from build123d import *

# Parameters (mm, degrees)
SCHNITT_LINEAR_AUSTRAGEN2_DEPTH = 7.5


with BuildPart() as part:
    # Skizze1 → Rotation1 (revolve)
    with BuildSketch(Plane.XY, mode=Mode.PRIVATE) as rotation1_sk:
        with BuildLine():
            Line((14.3, 4.8), (15.4, 4.8))
            Line((15.4, 4.8), (15.4, 5))
            Line((15.4, 5), (16.4, 5))
            Line((16.4, 5), (16.9, 4.5))
            Line((16.9, 4.5), (16.9, 0))
            Line((16.9, 0), (-12.3, 0))
            Line((-12.3, 0), (-12.3, 5))
            Line((-12.3, 5), (-3.05, 5))
            Line((-3.05, 5), (-3.05, 4.25))
            Line((-3.05, 4.25), (-2.3, 4.25))
            Line((-2.3, 4.25), (-2.3, 7.5))
            Line((-2.3, 7.5), (-0.7, 7.5))
            Line((-0.7, 7.5), (-0.7, 5.3))
            ThreePointArc((-0.7, 5.3), (-0.612132034, 5.087867966), (-0.4, 5))
            Line((-0.4, 5), (14.3, 5))
            Line((14.3, 5), (14.3, 4.8))
        make_face()
    revolve(rotation1_sk.sketch.rotate(Axis((-55.671450842, 0, 0), (1, 0, 0)), 90), axis=Axis((-55.671450842, 0, 0), (1, 0, 0)))

    # Skizze5 → Schnitt-Linear austragen2 (cut, symmetric)
    with BuildSketch(Plane(origin=(0, 0, 0), x_dir=(0, 0, -1), z_dir=(1, 0, 0))):
        with BuildLine():
            Line((-3.741657387, 6.5), (3.741657387, 6.5))
            ThreePointArc((3.741657387, 6.5), (0, 7.5), (-3.741657387, 6.5))
        make_face()
        with BuildLine():
            Line((-3.741657387, -6.5), (3.741657387, -6.5))
            ThreePointArc((3.741657387, -6.5), (0, -7.5), (-3.741657387, -6.5))
        make_face()
    extrude(amount=SCHNITT_LINEAR_AUSTRAGEN2_DEPTH, both=True, mode=Mode.SUBTRACT)


solid = part.part
Source: CAD feature listing. Evaluate the final solid. Frame: model axes, mm. A direction names the side the tool comes from. Give positions to 0.01 mm unless a question says otherwise; leave off trailing zeros. Write each loop counter-clockwise with the first axis right and the second up, starting at its lowest first coordinate (ties: lowest second). Pieces come first, ordered by that corner, then holes. Notation, with made-up numbers: M 49.25,74.5 L 106.25,74.5 A16 ccw 106.25,96.5 Z; hole C -28,10.5 d7. An arc over 180 degrees is marked long. Return JSON: item names as keys, results as strings. Group by question number.
1) Set-up query: faces 1 (the face through (-1.5, -0.1, -7.5)), 2 (the face through (-2.3, -4.4, 0.1)), 3 (the face through (7, 0, -5)). Return all of +Z, -Z, +X, -X, +Y, -Y with unobstructed straight access to the full face (end or side cutting, diameter ignored); none if empty.
2) Cut plane B-B, the plane x = 4. Output: boundary loops of the cut face in (y, z).
3) Ray query, L1, parallel to X at y = -6, z = -3.5; L2, parallel to Y at x = -10.25, z = 0; L3, parallel to X at y = -4, z = -2.75. Return the intervals inside material, ascending.
4) Draft query along X for faces 4 (the face through (16.9, 0, 0)), 5 (the face through (-12.3, 0, 0)), 6 (the face through (14.86, -4.05, 2.58)), 7 (the face through (-8, 0, -5)). Return one class per face: released by +X, released by -X, zero draft, split by the parting line, or undercut.
5) First-contact query: pin 1 Ø3 at (x, y) = (5, -4.5) entering from +Z; pin 2 Ø5 at (x, z) = (3, -5.5) entering from -Y; pin 3 Ø1.5 at (x, y) = (5.5, -3.5) entering from -Z. Flat tips, straight axial feed; report the tip coordinate or a pass-through.
6) Cut plane C-C, the plane x = -1.5. Output: boundary loops of the cut face in (y, z), then the cut area to 3 significant figures.
7) Cut plane A-A, the plane z = 0. Output: boundary loops of the cut face in (x, y), then the cut area to 3 significant figures.
Data:
{
 "1": {"face 1": "-Z, +X, -X", "face 2": "none", "face 3": "+X"},
 "2": {"outline": "C 0,0 d10"},
 "3": {"L1": "x = -2.3 to -0.7", "L2": "y = -5 to 5", "L3": "x = -12.3 to -3.05, -2.3 to 14.3, 15.4 to 16.55"},
 "4": {"face 4": "released by +X", "face 5": "released by -X", "face 6": "undercut", "face 7": "zero draft"},
 "5": {"pin 1": "stops at z = 4", "pin 2": "stops at y = -4", "pin 3": "stops at z = -4.18"},
 "6": {"outline": "M -6.5,-3.74 A7.5 ccw 6.5,-3.74 L 6.5,3.74 A7.5 ccw -6.5,3.74 Z", "area": "167 mm²"},
 "7": {"outline": "M -12.3,-5 L -3.05,-5 L -3.05,-4.25 L -2.3,-4.25 L -2.3,-6.5 L -0.7,-6.5 L -0.7,-5.3 A0.3 cw -0.4,-5 L 14.3,-5 L 14.3,-4.8 L 15.4,-4.8 L 15.4,-5 L 16.4,-5 L 16.9,-4.5 L 16.9,4.5 L 16.4,5 L 15.4,5 L 15.4,4.8 L 14.3,4.8 L 14.3,5 L -0.4,5 A0.3 cw -0.7,5.3 L -0.7,6.5 L -2.3,6.5 L -2.3,4.25 L -3.05,4.25 L -3.05,5 L -12.3,5 Z", "area": "295 mm²"}
}
